Build history of the part. All positions in model axes, mm. A direction names the side the tool comes from. Round coordinates to 2 decimals unless told otherwise and drop trailing zeros. Loops run counter-clockwise (first coordinate to the right, second up) from the corner with the lowest first, then second, coordinate; pieces in that order, holes last. Notation, with made-up numbers: (41.5, 55) - (89.5, 55) arc R21 ccw to (89.5, 79) - close; hole circle Ø9 at (4, 59). An arc over 180 degrees is marked (long way). Use one line per item in the form item = value. Start each with the question number.
Q1. Saw through at B-B (y = 0.5). Give the cut face in (x, z).
Q2. Pin check, flat tips, straight feed: pin 1 (3 mm diameter, centred on x = -12.25, z = 0, fed in from -Y); pin 2 (4 mm diameter, centred on x = -5, y = -5, fed in from -Z); pin 3 (4 mm diameter, centred on x = 4, z = 1, fed in from -Y); pin 4 (0.5 mm diameter, centred on x = 7.5, z = 0, fed in from +Y). Stop position of each tip, or through.
Q3. Mould opens along Z. For faces 4 (the face through (4, 0, 0)), 5 (the face through (-5.097, -3.451, -0.163)), 6 (the face through (1.75, -3, 0)), 7 (the face through (7, 1, 0)) say: released by +Z, released by -Z, zero draft, split by the parting line, or undercut.
Q4. 3-axis set-ups, long thin cutter, end or side, ignore diameter. For faces 1 (the face through (3.5, 5, 0.1)), 2 (the face through (-3, 0, 1)), 3 (the face through (8.25, 2.97, -0.04)): which of +Z, -Z, +X, -X, +Y, -Y reach the whole face in a straight line?
Q5. Saw through at D-D (z = 0). Count the separate pieces of the cut face and the enclosed holes in it, then the cut area to 3 significant figures.
Q6. Saw through at C-C (x = -2). Give the cut face in (y, z).
Q7. Saw through at A-A (y = 3). Give the cut face in (x, z), then the cut area to 3 significant figures.
Q8. Drill centre lines: line 1 (X direction, y = 3.5, z = 0); line 2 (X direction, y = 2, z = -1.25); line 3 (Z direction, x = 0, y = -3). Where is each one in solid material? Low to high.
Autodesk Inventor part; units mm, degrees
ref_plane "YZ Plane" through (0, 0, 0) normal (1, 0, 0) x (0, 1, 0)
ref_plane "XZ Plane" through (0, 0, 0) normal (0, 1, 0) x (-1, 0, 0)
ref_plane "XY Plane" through (0, 0, 0) normal (0, 0, 1) x (1, 0, 0)
sketch "スケッチ1" plane through (0, 0, 0) normal (0, 1, 0) x (-1, 0, 0)
  arc A0 (-1.75, -3.0311) -> (-1.75, 3.0311) centre (0, 0) ccw
  arc A1 (-3.35, -3.8455) -> (-3.35, 3.8455) centre (0, 0) ccw
  line L0 (-1.75, 3.0311) -> (-1.75, -3.0311)
  line L1 (-3.35, 3.8455) -> (-3.35, -3.8455)
  point P0 (-1.75, 0)
  point P1 (3.5, 0)
  dimension "d0" = 7
  dimension "d1" = 1.6
  dimension "d3" = 1.6
  dimension "d21" = 5.25
extrude "押し出し1" add sketch "スケッチ1" against normal blind 7
sketch "スケッチ2" plane through (0, 0, 0) normal (0, 1, 0) x (-1, 0, 0)
  circle A0 centre (0, 0) radius 3
  circle A1 centre (7.25, 0) radius 1
  circle A2 centre (12.25, 0) radius 1
  line L0 (21.35, 0) -> (-16.3472, 0)
  line L1 (-21.4194, 0) -> (25.6478, 0)
  line L2 (0, 13.6596) -> (0, -18.5916)
  circle A3 centre (-7.25, 0) radius 1
  circle A4 centre (-12.25, 0) radius 1
  arc A5 (13.1684, -2.3252) -> (13.1684, 2.3252) centre (12.25, 0) ccw
  line L3 (13.1684, 2.3252) -> (2.5714, 6.5106)
  line L4 (13.1684, -2.3252) -> (2.5714, -6.5106)
  arc A6 (-13.1684, 2.3252) -> (-13.1684, -2.3252) centre (-12.25, 0) ccw
  line L5 (-13.1684, 2.3252) -> (-2.5714, 6.5106)
  line L6 (-13.1684, -2.3252) -> (-2.5714, -6.5106)
  arc A7 (-2.5714, -6.5106) -> (2.5714, -6.5106) centre (0, 0) ccw
  arc A8 (2.5714, 6.5106) -> (-2.5714, 6.5106) centre (0, 0) ccw
  circle A9 centre (0, 0) radius 5.5
  circle A10 centre (0, 0) radius 6.5
  dimension "d6" = 6
  dimension "d7" = 7.25
  dimension "d8" = 5
  dimension "d9" = 2
  dimension "d11" = 5
  dimension "d12" = 7
  dimension "d17" = 11
  dimension "d18" = 13
extrude "押し出し2" add sketch "スケッチ2" along normal blind 1 contours L0 A9 L2 A0 | A0 L2 A9 L0 | A0 L0 A9 L2 | L2 A9 L0 A0 | A9 L2 A10 A1 L0 | L0 A1 A10 L2 A9 | A9 L0 A3 A10 L2 | L2 A10 A3 L0 A9 | L0 A10 A1 | A1 A10 L0 | A10 A3 L0 A4 A6 L5 A8 L2 | L2 A8 L3 A5 L0 A2 A1 A10 | A10 A1 L0 A2 A5 L4 A7 L2 | L2 A7 L6 A6 L0 A4 A3 A10 | A1 L0 A10 | A10 L0 A1 | A3 A10 L0 | L0 A10 A3 | A10 L0 A3 | A3 L0 A10 | L0 A2 | A2 L0 | A4 L0 | L0 A4
extrude "押し出し3" add sketch "スケッチ2" along normal blind 5 contours L0 A9 L2 A0 | A0 L2 A9 L0 | A0 L0 A9 L2 | L2 A9 L0 A0 | A9 L2 A10 A1 L0 | L0 A1 A10 L2 A9 | A9 L0 A3 A10 L2 | L2 A10 A3 L0 A9 | A10 A3 L0 A4 A6 L5 A8 L2 | L2 A8 L3 A5 L0 A2 A1 A10 | A10 A1 L0 A2 A5 L4 A7 L2 | L2 A7 L6 A6 L0 A4 A3 A10
extrude "押し出し4" cut sketch "スケッチ2" along normal blind 4 contours A9 L2 A10 A1 L0 | L0 A1 A10 L2 A9 | A9 L0 A3 A10 L2 | L2 A10 A3 L0 A9 | L0 A10 A1 | A1 A10 L0 | A3 A10 L0 | L0 A10 A3 picked at (6.3418, -0.0745) picked at (6.3418, 0.0745) picked at (-6.3418, -0.0745) picked at (-6.3418, 0.0745)
properties part number "stick"
Report:
q1.outline = (-13.17, -2.33) - (-2.57, -6.51) arc R7 ccw to (2.57, -6.51) - (13.17, -2.33) arc R2.5 ccw to (13.17, 2.33) - (2.57, 6.51) arc R7 ccw to (-2.57, 6.51) - (-13.17, 2.33) arc R2.5 ccw to start; circle Ø11 at (0, 0); hole circle Ø13 at (0, 0); hole circle Ø6 at (0, 0)
q2.pin_1 = 0
q2.pin_2 = -4.12
q2.pin_3 = -7
q2.pin_4 = 1
q3.face_4 = zero draft
q3.face_5 = split by the parting line
q3.face_6 = undercut
q3.face_7 = undercut
q4.face_1 = +Z, -Z, +X, -X, +Y
q4.face_2 = -Y
q4.face_3 = +Y
q5.separate_pieces = 4
q5.enclosed_holes = 0
q5.area = 101 mm²
q6.outline = (-7, -4.69) - (0, -4.69) - (0, -5.12) - (4, -5.12) - (4, -6.18) - (0, -6.18) - (0, -6.71) - (5, -6.71) - (5, -2.24) - (0, -2.24) - (0, -2.87) - (-7, -2.87) - close; (-7, 2.87) - (0, 2.87) - (0, 2.24) - (5, 2.24) - (5, 6.71) - (0, 6.71) - (0, 6.18) - (4, 6.18) - (4, 5.12) - (0, 5.12) - (0, 4.69) - (-7, 4.69) - close
q7.outline = (-13.17, -2.33) - (-2.57, -6.51) arc R7 ccw to (2.57, -6.51) - (13.17, -2.33) arc R2.5 ccw to (13.17, 2.33) - (2.57, 6.51) arc R7 ccw to (-2.57, 6.51) - (-13.17, 2.33) arc R2.5 ccw to start; circle Ø11 at (0, 0); hole circle Ø2 at (-12.25, 0); hole (-6.47, -0.63) arc R6.5 ccw to (6.47, -0.63) arc R1 ccw (long way) to (6.47, 0.63) arc R6.5 ccw to (-6.47, 0.63) arc R1 ccw (long way) to start; hole circle Ø6 at (0, 0); hole circle Ø2 at (12.25, 0)
q7.area = 190 mm²
q8.line_1 = -14.75 to -13.25, -11.25 to -8.25, -5.5 to -3, 3 to 5.5, 8.25 to 11.25, 13.25 to 14.75
q8.line_2 = -14.42 to -6.38, -5.36 to -2.73, 2.73 to 5.36, 6.38 to 14.42
q8.line_3 = -5.1 to -3.5, 3.5 to 5.1
